from build123d import *

# Parameters (mm, degrees)
F0_W     = 1200
F0_H     = 360
F1_DEPTH = 250
F2_R     = 60
F3_DEPTH = 250.001
F4_R     = 300
F5_DEPTH = 275
F6_R     = 200
F7_DEPTH = 150
F8_R     = 100
F9_DEPTH = 400.001
F10_R    = 100


with BuildPart() as f1:
    # F0 (on Top) → F1 (new body)
    with BuildSketch(Plane.XY):
        Rectangle(F0_W, F0_H)
    extrude(amount=F1_DEPTH)

    # F2 (on face) → F3 (cut, through all)
    with BuildSketch(Plane.XY.offset(250)):
        with Locations((-456.190459, 0)):
            Circle(F2_R)
        with Locations((443.809541, 0)):
            Circle(F2_R)
    extrude(amount=-F3_DEPTH, mode=Mode.SUBTRACT)

    # F4 (on face) → F5 (join, symmetric)
    with BuildSketch(Plane.XY.offset(250)):
        Circle(F4_R)
        with BuildLine():
            ThreePointArc((240, -180), (284.604989, -94.86833), (300, 0))
            ThreePointArc((300, 0), (284.604989, 94.86833), (240, 180))
            Line((240, 180), (-240, 180))
            ThreePointArc((-240, 180), (-300, 0), (-240, -180))
            Line((-240, -180), (240, -180))
        make_face()
    extrude(amount=F5_DEPTH, both=True)

    # F6 (on face) → F7 (cut)
    with BuildSketch(Plane.XY.offset(525)):
        Circle(F6_R)
    extrude(amount=-F7_DEPTH, mode=Mode.SUBTRACT)

    # F8 (on face) → F9 (cut, through all)
    with BuildSketch(Plane.XY.offset(375)):
        Circle(F8_R)
    extrude(amount=-F9_DEPTH, mode=Mode.SUBTRACT)

    # F10
    f10_edges = [f1.edges().sort_by_distance(p)[0] for p in [
        (600, -180, 125),
        (600, 180, 125),
        (-600, -180, 125),
        (-600, 180, 125),
    ]]
    fillet(f10_edges, radius=F10_R)


solid = f1.part
Work out the finished part from the listing and answer in its coordinate system (mm). A direction names the side the tool comes from. Coordinates: 2 decimals unless noted, no trailing zeros. Write each loop counter-clockwise with the first axis right and the second up, starting at its lowest first coordinate (ties: lowest second). Pieces come first, ordered by that corner, then holes. Notation, with made-up numbers: (22, 74) - (61, 74) arc R33 ccw to (61, 102) - close; hole circle Ø5 at (67, 69.25). An arc over 180 degrees is marked (long way). One line per question, with ' | ' between items.
1) The mould has two halves that part along Y. Classify faces 1 (the face through (-398.96, 18.02, 126.75)), 2 (the face through (377, 3, 0)), 3 (the face through (-569.929, -151.484, 126.75)): +Y half, -Y half, draft (parallel to the pull), parting line (faces both ways), or undercut.
Checks:
face 1: undercut | face 2: draft | face 3: -Y half
2) Find section D-D, the plane y = 159.5. Determine the outline of the cut face in (x, z), and give its area (3 significant figures).
Checks:
outline: (-560.66, 0) - (-254.09, 0) - (-254.09, -25) - (254.09, -25) - (254.09, 0) - (560.66, 0) - (560.66, 250) - (254.09, 250) - (254.09, 525) - (120.66, 525) - (120.66, 375) - (-120.66, 375) - (-120.66, 525) - (-254.09, 525) - (-254.09, 250) - (-560.66, 250) - close | area: 397,000 mm2
3) Find section B-B, the plane x = 0. Determine the outline of the cut face in (y, z), and give its area (3 significant figures).
Checks:
outline: (-300, -25) - (-100, -25) - (-100, 375) - (-200, 375) - (-200, 525) - (-300, 525) - close; (100, -25) - (300, -25) - (300, 525) - (200, 525) - (200, 375) - (100, 375) - close | area: 190,000 mm2
4) Find section C-C, the plane z = 88. Determine the outline of the cut face in (x, y).
Checks:
outline: (-600, -80) arc R100 ccw to (-500, -180) - (-240, -180) arc R300 ccw to (240, -180) - (500, -180) arc R100 ccw to (600, -80) - (600, 80) arc R100 ccw to (500, 180) - (240, 180) arc R300 ccw to (-240, 180) - (-500, 180) arc R100 ccw to (-600, 80) - close; hole circle Ø120 at (-456.19, 0); hole circle Ø200 at (0, 0); hole circle Ø120 at (443.81, 0)
5) Consider probe 1 along X at (y, z) = (4, 458); probe 2 along Y at (x, z) = (0, 57); probe 3 along Z at (x, y) = (315, -54.5). Determine where each line is inside the solid, lowest interval first. Write a range as [from, to].
Checks:
probe 1: [-299.97, -199.96], [199.96, 299.97] | probe 2: [-300, -100], [100, 300] | probe 3: [0, 250]
6) Flat-ended cylindrical pins translate along their axes: P1, Ø3, axis at x = -426, y = -63, coming from the +Z side; P2, Ø6, axis at y = 206, z = 36, coming from the +X side; P3, Ø3, axis at x = -109.5, z = 445.5, coming from the -Y side. Find the tip coordinate at first contact, or state that the pin passes through.
Checks:
P1: z = 250 | P2: x = 220.89 | P3: y = -279.89
7) Find section A-A, the plane y = 0. Determine the outline of the cut face in (x, z), and give its area (3 significant figures).
Checks:
outline: (-600, 0) - (-516.19, 0) - (-516.19, 250) - (-600, 250) - close; (-396.19, 0) - (-300, 0) - (-300, -25) - (-100, -25) - (-100, 375) - (-200, 375) - (-200, 525) - (-300, 525) - (-300, 250) - (-396.19, 250) - close; (100, -25) - (300, -25) - (300, 0) - (383.81, 0) - (383.81, 250) - (300, 250) - (300, 525) - (200, 525) - (200, 375) - (100, 375) - close; (503.81, 0) - (600, 0) - (600, 250) - (503.81, 250) - close | area: 280,000 mm2
8) For faces 4 (the face through (-92, -42, 375)), 5 (the face through (368, 180, 123)), 6 (the face through (-372, -180, 123)), 7 (the face through (368, -180, 123)), determine the directions among +Z, -Z, +X, -X, +Y, -Y from which every point of the face is accessible in a straight line to the end or side of a thin tool.
Checks:
face 4: +Z | face 5: +Z, -Z, +X, +Y | face 6: +Z, -Z, -X, -Y | face 7: +Z, -Z, +X, -Y
